Study the drawing (mm; zero at the part's minimum x, y, z) and answer. Coordinates: 2 decimals unless noted, no trailing zeros. Put each result on its own line as item: value.
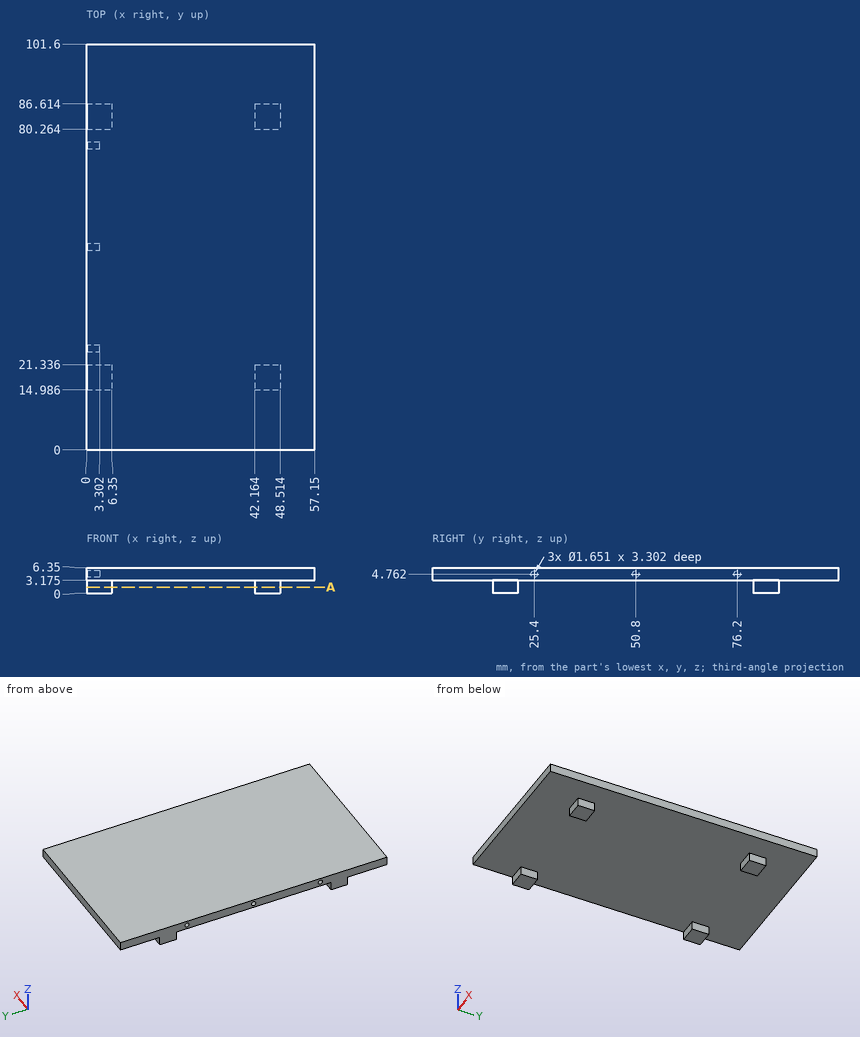
Q1. Given pin 1 (6 mm diameter, centred on x = 43, y = 10.5, fed in from -Z) (1 decimal); pin 2 (2.5 mm diameter, centred on y = 19, z = 1.5, fed in from +X); pin 3 (1 mm diameter, centred on x = 5, z = 1.5, fed in from -Y), each flat-ended and moving along its own axis, determine where each tip first touches the part or whether it passes through.
Answers below:
pin 1: stops at z = 3.2
pin 2: stops at x = 48.51
pin 3: stops at y = 14.99
Q2. Find section A-A on z = 1.5. Give the number of separate pieces and of enclosed holes in the cut face, plus the area to 3 significant figures.
Answers below:
separate pieces: 4
enclosed holes: 0
area: 161 mm^2
Q3. Consider line 1 along Y through (x, z) = (44, 2) (1 decimal); line 2 along X through (y, z) = (26, 4.25). Determine where each line is inside the solid, lowest interval first.
Answers below:
line 1: y = 15 to 21.3, 80.3 to 86.6
line 2: x = 3.3 to 57.15
